from build123d import *

# Parameters (mm, degrees)
SKETCH_1_R                                       = 19
HORN_FLANGE_D38_DEPTH                            = 4
SKETCH_2_R                                       = 14
SHAFT_CLAMP_HUB_DEPTH                            = 16
SHAFT_D5P2_DEPTH                                 = 32.272991542
SHAFT_D5P2_DEPTH_BACK                            = 32.272991542
SKETCH_3_R                                       = 2.6
CLAMP_SPLIT_DEPTH                                = 32.272991542
CLAMP_SPLIT_DEPTH_BACK                           = 32.272991542
SKETCH_4_W                                       = 1.2
SKETCH_4_H                                       = 17.8
HORN_TWO_ADJUSTMENT_SLOTS_VERIFY_HORN_DEPTH      = 32.272991542
HORN_TWO_ADJUSTMENT_SLOTS_VERIFY_HORN_DEPTH_BACK = 32.272991542
SKETCH_5_W                                       = 4.5
SKETCH_5_H                                       = 2.6
COUPLER_CLAMP_M3_DEPTH                           = 32.272991542
COUPLER_CLAMP_M3_DEPTH_BACK                      = 32.272991542
SKETCH_6_R                                       = 1.7


with BuildPart() as part:
    # 草图1 → Horn_flange_D38 (new body)
    with BuildSketch(Plane.XY):
        Circle(SKETCH_1_R)
    extrude(amount=HORN_FLANGE_D38_DEPTH)

    # 草图2 → Shaft_clamp_hub (add)
    with BuildSketch(Plane.XY):
        Circle(SKETCH_2_R)
    extrude(amount=SHAFT_CLAMP_HUB_DEPTH)

    # 草图3 → Shaft_D5p2 (cut, two sides: drawn at the far end of the back side and taken through both)
    with BuildSketch(Plane.XY.offset(-SHAFT_D5P2_DEPTH_BACK)):
        Circle(SKETCH_3_R)
    extrude(amount=SHAFT_D5P2_DEPTH + SHAFT_D5P2_DEPTH_BACK, mode=Mode.SUBTRACT)

    # 草图4 → Clamp_split (cut, two sides: drawn at the far end of the back side and taken through both)
    with BuildSketch(Plane.XY.offset(-CLAMP_SPLIT_DEPTH_BACK)):
        with Locations((0, 11.1)):
            Rectangle(SKETCH_4_W, SKETCH_4_H)
    extrude(amount=CLAMP_SPLIT_DEPTH + CLAMP_SPLIT_DEPTH_BACK, mode=Mode.SUBTRACT)

    # 草图5 → Horn_two_adjustment_slots_VERIFY_HORN (cut, two sides: drawn at the far end of the back side and taken through both)
    with BuildSketch(Plane.XY.offset(-HORN_TWO_ADJUSTMENT_SLOTS_VERIFY_HORN_DEPTH_BACK)):
        with Locations((-8.25, 0)):
            Rectangle(SKETCH_5_W, SKETCH_5_H)
        with Locations((8.25, 0)):
            Rectangle(SKETCH_5_W, SKETCH_5_H)
    extrude(amount=HORN_TWO_ADJUSTMENT_SLOTS_VERIFY_HORN_DEPTH + HORN_TWO_ADJUSTMENT_SLOTS_VERIFY_HORN_DEPTH_BACK, mode=Mode.SUBTRACT)

    # 草图6 → Coupler_clamp_M3 (cut, two sides: drawn at the far end of the back side and taken through both)
    with BuildSketch(Plane(origin=(0, 0, 0), x_dir=(0, 0, -1), z_dir=(1, 0, 0)).offset(-COUPLER_CLAMP_M3_DEPTH_BACK)):
        with Locations((-10, 9)):
            Circle(SKETCH_6_R)
    extrude(amount=COUPLER_CLAMP_M3_DEPTH + COUPLER_CLAMP_M3_DEPTH_BACK, mode=Mode.SUBTRACT)


solid = part.part
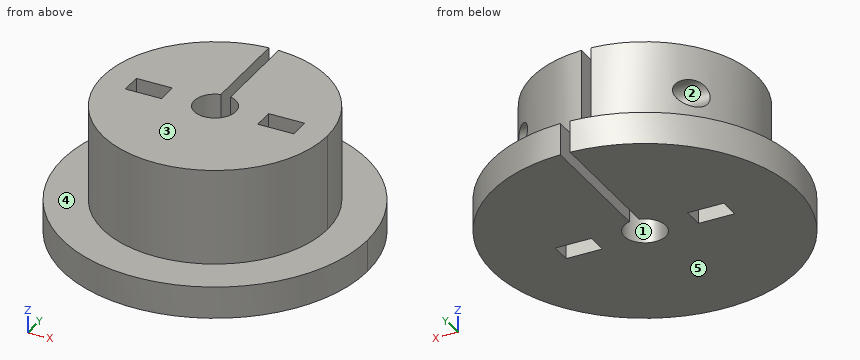
Input: part model. Units: mm. Frame: model coordinates. Face numbers are marked on the shaded views. A direction names the side the tool comes from. Give positions to 0.01 mm unless a question says otherwise; leave off trailing zeros. Write each loop counter-clockwise with the first axis right and the second up, starting at its lowest first coordinate (ties: lowest second). Pieces come first, ordered by that corner, then holes.
Q1. Section B-B, the plane x = -9. Output: boundary loops of the cut face in (y, z), plus the area to 3 significant figures.
Q2. Section A-A, the plane z = 1.5. Output: boundary loops of the cut face in (x, y), plus the area to 3 significant figures.
Q3. First-contact query: P1, Ø3.5, axis at x = -8.5, z = 6.5, coming from the -Y side; P2, Ø0.8, axis at y = 0.5, z = 4.5, coming from the -X side; P3, Ø4, axis at x = -7, z = 9, coming from the -Y side. Flat tips, straight axial feed; report the tip coordinate or a pass-through.
Q4. Set-up query: the marked faces 4 and 5. Return all of +Z, -Z, +X, -X, +Y, -Y with unobstructed straight access to the full face (end or side cutting, diameter ignored); none if empty.
Q5. Pull-direction query (Z, two-part tool) for the marked faces 1, 2 and 3; classes: pulls with the +Z half, pulls with the -Z half, needs draft (parallel to the pull), parting line crosses it, or undercut.
Q6. Section D-D, the plane y = 4. Output: boundary loops of the cut face in (x, z).
Q7. Material intervals for probe 1 along X at (y, z) = (0, 5.25); probe 2 along Z at (x, y) = (-5, 9); probe 3 along Y at (x, z) = (9.5, 7), sorted ascending.
Q8. Section C-C, the plane z = 9. Output: boundary loops of the cut face in (x, y).
Filled in:
1. outline: (-16.73, 0) - (-1.3, 0) - (-1.3, 16) - (-10.72, 16) - (-10.72, 4) - (-16.73, 4) - close; (1.3, 0) - (16.73, 0) - (16.73, 4) - (10.72, 4) - (10.72, 16) - (1.3, 16) - close; hole circle Ø3.4 at (9, 10)
1. area: 341 mm2
2. outline: (-0.6, 2.53) - (-0.6, 18.99) arc R19 ccw (long way) to (0.6, 18.99) - (0.6, 2.53) arc R2.6 cw (long way) to start; hole (-10.5, -1.3) - (-6, -1.3) - (-6, 1.3) - (-10.5, 1.3) - close; hole (6, -1.3) - (10.5, -1.3) - (10.5, 1.3) - (6, 1.3) - close
2. area: 1,070 mm2
3. P1: stops at y = -12.27
3. P2: stops at x = -14
3. P3: stops at y = -13.08
4. face 4: +Z
4. face 5: -Z, +X, -X, +Y, -Y
5. face 1: needs draft
5. face 2: undercut
5. face 3: pulls with the +Z half
6. outline: (-18.57, 0) - (-0.6, 0) - (-0.6, 16) - (-13.42, 16) - (-13.42, 4) - (-18.57, 4) - close; (0.6, 0) - (18.57, 0) - (18.57, 4) - (13.42, 4) - (13.42, 16) - (0.6, 16) - close
7. probe 1: x = -14 to -10.5, -6 to -2.6, 2.6 to 6, 10.5 to 14
7. probe 2: z = 0 to 8.3, 11.7 to 16
7. probe 3: y = -10.28 to -1.3, 1.3 to 10.28
8. outline: (-11.74, 7.63) arc R14 ccw (long way) to (11.74, 7.63) - (0.6, 7.63) - (0.6, 2.53) arc R2.6 cw (long way) to (-0.6, 2.53) - (-0.6, 7.63) - close; (-9.4, 10.37) - (-0.6, 10.37) - (-0.6, 13.99) arc R14 ccw to start; (0.6, 10.37) - (9.4, 10.37) arc R14 ccw to (0.6, 13.99) - close; hole (-10.5, -1.3) - (-6, -1.3) - (-6, 1.3) - (-10.5, 1.3) - close; hole (6, -1.3) - (10.5, -1.3) - (10.5, 1.3) - (6, 1.3) - close
